Design review of the part built by this model. Coordinates are the model's own, in mm. Face numbers are marked on the shaded views. A direction names the side the tool comes from. Coordinates: 2 decimals unless noted, no trailing zeros. Write each loop counter-clockwise with the first axis right and the second up, starting at its lowest first coordinate (ties: lowest second). Pieces come first, ordered by that corner, then holes.
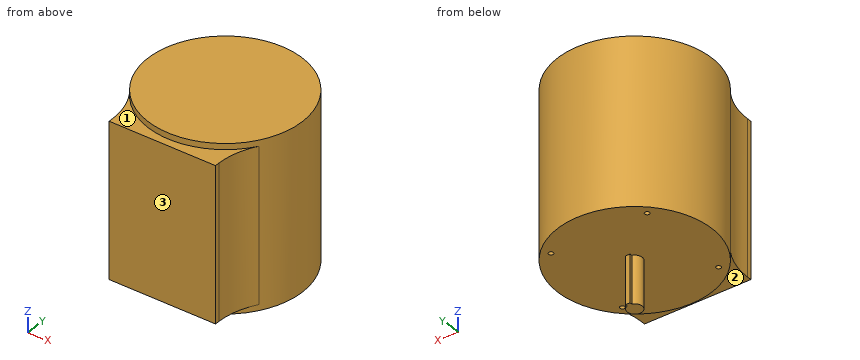
Autodesk Inventor part; units mm, degrees
ref_plane "YZ Plane" through (0, 0, 0) normal (1, 0, 0) x (0, 1, 0)
ref_plane "XY Plane" through (0, 0, 0) normal (0, 0, 1) x (1, 0, 0)
sketch "Sketch1" plane through (0, 0, 0) normal (0, 0, 1) x (1, 0, 0)
  circle A0 centre (0, 0) radius 7.9375
  line L0 (-2.4257, 7.5578) -> (-2.4257, 10.0978)
  line L1 (-2.4257, 10.0978) -> (2.4257, 10.0978)
  line L2 (2.4257, 10.0978) -> (2.4257, 7.5578)
  point P0 (0, 10.0978)
  dimension "d0" = 15.875
  dimension "d1" = 2.54
  dimension "d2" = 4.8514
extrude "Extrusion1" add sketch "Sketch1" along normal blind 50.8
sketch "Sketch2" plane through (0, 0, 50.8) normal (0, 0, 1) x (1, 0, 0)
  circle A0 centre (0, 0) radius 82.55
  dimension "d5" = 165.1
extrude "Extrusion2" add sketch "Sketch2" along normal blind 177.8
sketch "Sketch3" plane through (0, 0, 50.8) normal (0, 0, -1) x (-1, 0, 0)
  circle A0 centre (0, 0) radius 73.025
  arc A1 (-2.4257, 7.5578) -> (2.4257, 7.5578) centre (0, 0) ccw
  line L0 (0, 0) -> (51.6365, 51.6365)
  line L1 (0, 0) -> (73.025, 0) construction
  line L2 (0, 0) -> (51.6365, -51.6365)
  line L3 (0, 0) -> (73.025, 0) construction
  line L4 (0, 0) -> (-51.6365, 51.6365)
  line L5 (0, 0) -> (73.025, 0) construction
  line L6 (0, 0) -> (-51.6365, -51.6365)
  line L7 (0, 0) -> (73.025, 0) construction
  dimension "d8" = 146.05
  dimension "d9" = 45
  dimension "d10" = 45
  dimension "d11" = 135
  dimension "d12" = 135
hole "Hole1" at (51.6365, 51.6365, 50.8) at (-51.6365, 51.6365, 50.8) at (-51.6365, -51.6365, 50.8) at (51.6365, -51.6365, 50.8) direction (0, 0, 1) diameter 4.9784 depth 19.05 tip angle 118
ref_plane "Work Plane1" through (0, -82.55, 50.8) normal (0, 1, 0) x (-1, 0, 0)
sketch "Sketch4" plane through (0, -82.55, 50.8) normal (0, 1, 0) x (-1, 0, 0)
  line L0 (82.55, 177.8) -> (-82.55, 177.8)
  line L1 (-82.55, 0) -> (82.55, 0)
  line L2 (82.55, 0) -> (82.55, 177.8)
  line L3 (-82.55, 0) -> (-82.55, 177.8)
  line L4 (-57.15, 6.35) -> (57.15, 6.35)
  line L5 (57.15, 6.35) -> (57.15, 171.45)
  line L6 (57.15, 171.45) -> (-57.15, 171.45)
  line L7 (-57.15, 171.45) -> (-57.15, 6.35)
  point P0 (0, -50.8)
  point P1 (0, 6.35)
  dimension "d20" = 165.1
  dimension "d21" = 6.35
  dimension "d22" = 114.3
extrude "Extrusion3" add sketch "Sketch4" along normal blind 25.4 and the other way blind 8.4074 contours L7 L6 L5 L4
fillet "Fillet1" radius 76.2 1 edges at (-57.15, -59.5683, 139.7)
fillet "Fillet2" radius 76.2 1 edges at (57.15, -59.5683, 139.7)
equation "\"d3\" = ShaftL"
equation "\"d5\" = MotoD"
equation "\"d6\" = MotoL"
equation "\"ShaftL\" = 50.8"
equation "\"MotoD\" = 165.1"
equation "\"MotoL\" = 177.8"
properties part number "oldMotor4"
(1) Consider section B-B (z = 212). Give the boundary of the cut face in (x, y), plus the area to 3 significant figures.
(2) Consider section C-C (y = -72). Give the boundary of the cut face in (x, z), plus the area to 3 significant figures.
(3) Consider section D-D (z = 42.5). Give the boundary of the cut face in (x, y) (1 decimal), plus the area to 3 significant figures.
(4) Insertion check: pin 1 Ø4 at (x, y) = (51.64, -51.64) entering from -Z; pin 2 Ø1.3 at (y, z) = (9.5, 33) entering from +X; pin 3 Ø23 at (x, y) = (6.5, -71.5) entering from -Z. Each pin has a flat end and moves straight along its axis. Give the tip position at first contact, or say it passes through.
(5) For the marked faces 1, 2 and 3, list the 3-axis set-ups (+Z, -Z, +X, -X, +Y, -Y) from which the entire face can be reached by the end or side of a thin tool; tool diameter is ignored.
(6) Wall thickness on line 1 (Z direction, x = 47, y = 19); line 2 (X direction, y = -2.5, z = 52.5); line 3 (X direction, y = -3.5, z = 35): over which ranges is each line inside the solid? List them lowest first.
(7) Consider section A-A (y = 0). Give the boundary of the cut face in (x, z), plus the area to 3 significant figures.
Results:
1. outline: (-69.34, -44.79) arc R76.2 cw to (-57.15, -86.14) - (-57.15, -90.96) - (57.15, -90.96) - (57.15, -86.14) arc R76.2 cw to (69.34, -44.79) arc R82.55 ccw (long way) to start
1. area: 23,300 mm2
2. outline: (-58.47, 57.15) - (-40.38, 57.15) - (-40.38, 50.8) - (40.38, 50.8) - (40.38, 57.15) - (58.47, 57.15) - (58.47, 222.25) - (40.38, 222.25) - (40.38, 228.6) - (-40.38, 228.6) - (-40.38, 222.25) - (-58.47, 222.25) - close
2. area: 20,300 mm2
3. outline: (-2.4, 7.6) arc R7.9 ccw (long way) to (2.4, 7.6) - (2.4, 10.1) - (-2.4, 10.1) - close
3. area: 209 mm2
4. pin 1: stops at z = 70.14
4. pin 2: stops at x = 2.43
4. pin 3: stops at z = 50.8
5. face 1: +Z, -Y
5. face 2: -Z, -Y
5. face 3: +Z, -Z, +X, -X, -Y
6. line 1: z = 50.8 to 228.6
6. line 2: x = -82.51 to 82.51
6. line 3: x = -7.12 to 7.12
7. outline: (-82.55, 50.8) - (-7.94, 50.8) - (-7.94, 0) - (7.94, 0) - (7.94, 50.8) - (82.55, 50.8) - (82.55, 228.6) - (-82.55, 228.6) - close
7. area: 30,200 mm2
